from build123d import *

# Parameters (mm, degrees)
SKETCH1_R           = 1.5
SKETCH1_W           = 14
SKETCH1_H           = 14
BOSS_EXTRUDE1_DEPTH = 1.6
CUT_EXTRUDE1_DEPTH  = 1.6
FILLET1_R           = 3
SKETCH3_W           = 5.928661094
SKETCH3_H           = 12.435728147
SKETCH3_W_2         = 5.350255133
SKETCH3_H_2         = 5.928661094
SKETCH3_W_3         = 5.639458113
SKETCH3_W_4         = 6.651668543
SKETCH3_H_3         = 7.446976739
SKETCH3_W_5         = 5.928661093
SKETCH3_H_4         = 5.784059603
SKETCH3_H_5         = 4.627247683
BOSS_EXTRUDE2_DEPTH = 1.6
CUT_EXTRUDE2_DEPTH  = 95.202490958
FILLET2_R           = 3
CUT_EXTRUDE3_DEPTH  = 95.202490958
FILLET3_R           = 3
FILLET4_R           = 3
FILLET7_R           = 2


with BuildPart() as part:
    # Sketch1 → Boss-Extrude1 (new body)
    with BuildSketch(Plane.XY):
        with BuildLine():
            Line((69.256483633, 39.154946315), (-80.703110167, 39.058787515))
            ThreePointArc((-80.703110167, 39.058787515), (-82.819785745, 38.18282616), (-83.701171171, 36.068403419))
            Line((-83.701171171, 36.068403419), (-83.931946571, -35.933513481))
            ThreePointArc((-83.931946571, -35.933513481), (-83.056679124, -38.061046878), (-80.931961975, -38.943128786))
            Line((-80.931961975, -38.943128786), (-34.162352475, -38.943128786))
            ThreePointArc((-34.162352475, -38.943128786), (-34.036703471, -38.945761219), (-33.911274976, -38.953653901))
            Line((-33.911274976, -38.953653901), (11.083089424, -42.732603701))
            ThreePointArc((11.083089424, -42.732603701), (11.20851792, -42.740496382), (11.334166924, -42.743128815))
            Line((11.334166924, -42.743128815), (59.596129524, -42.743128815))
            ThreePointArc((59.596129524, -42.743128815), (61.35026035, -42.176855395), (62.442179406, -40.69181219))
            Line((62.442179406, -40.69181219), (72.104457106, -11.70497919))
            ThreePointArc((72.104457106, -11.70497919), (72.219669608, -11.236842575), (72.258407243, -10.756295796))
            Line((72.258407243, -10.756295796), (72.258407243, 36.154946904))
            ThreePointArc((72.258407243, 36.154946904), (71.379047386, 38.276947252), (69.256483633, 39.154946315))
        make_face()
        with Locations((35.108407229, 34.256871219)):
            Circle(SKETCH1_R, mode=Mode.SUBTRACT)
        with Locations((-28.161592771, -22.743128781)):
            Circle(SKETCH1_R, mode=Mode.SUBTRACT)
        with Locations((-1.491592771, -27.493128781)):
            Circle(SKETCH1_R, mode=Mode.SUBTRACT)
        with Locations((-79.366592771, -9.443128781)):
            Circle(SKETCH1_R, mode=Mode.SUBTRACT)
        with Locations((49.358407229, -9.443128781)):
            Circle(SKETCH1_R, mode=Mode.SUBTRACT)
        with Locations((-59.891592771, 17.156871219)):
            Circle(SKETCH1_R, mode=Mode.SUBTRACT)
        with Locations((2.808407229, 28.556871219)):
            Rectangle(SKETCH1_W, SKETCH1_H, mode=Mode.SUBTRACT)
        with Locations((21.808407229, 28.556871219)):
            Rectangle(SKETCH1_W, SKETCH1_H, mode=Mode.SUBTRACT)
        with Locations((-35.191592771, 28.556871219)):
            Rectangle(SKETCH1_W, SKETCH1_H, mode=Mode.SUBTRACT)
        with Locations((-16.191592771, 28.556871219)):
            Rectangle(SKETCH1_W, SKETCH1_H, mode=Mode.SUBTRACT)
        with Locations((-70.816592771, 9.556871219)):
            Rectangle(SKETCH1_W, SKETCH1_H, mode=Mode.SUBTRACT)
        with Locations((-49.441592771, 9.556871219)):
            Rectangle(SKETCH1_W, SKETCH1_H, mode=Mode.SUBTRACT)
        with Locations((-30.441592771, 9.556871219)):
            Rectangle(SKETCH1_W, SKETCH1_H, mode=Mode.SUBTRACT)
        with Locations((-11.441592771, 9.556871219)):
            Rectangle(SKETCH1_W, SKETCH1_H, mode=Mode.SUBTRACT)
        with Locations((-39.941592771, -9.443128781)):
            Rectangle(SKETCH1_W, SKETCH1_H, mode=Mode.SUBTRACT)
        with Locations((-1.941592771, -9.443128781)):
            Rectangle(SKETCH1_W, SKETCH1_H, mode=Mode.SUBTRACT)
        with Locations((26.558407229, 9.556871219)):
            Rectangle(SKETCH1_W, SKETCH1_H, mode=Mode.SUBTRACT)
        with Locations((36.058407229, -9.443128781)):
            Rectangle(SKETCH1_W, SKETCH1_H, mode=Mode.SUBTRACT)
        with Locations((17.508407229, -32.243128781)):
            Rectangle(SKETCH1_W, SKETCH1_H, mode=Mode.SUBTRACT)
        with Locations((-70.816592771, -28.443128781)):
            Rectangle(SKETCH1_W, SKETCH1_H, mode=Mode.SUBTRACT)
        with Locations((-73.191592771, 28.556871219)):
            Rectangle(SKETCH1_W, SKETCH1_H, mode=Mode.SUBTRACT)
        with Locations((-54.191592771, 28.556871219)):
            Rectangle(SKETCH1_W, SKETCH1_H, mode=Mode.SUBTRACT)
        with Locations((7.558407229, 9.556871219)):
            Rectangle(SKETCH1_W, SKETCH1_H, mode=Mode.SUBTRACT)
        with Locations((-66.066592771, -9.443128781)):
            Rectangle(SKETCH1_W, SKETCH1_H, mode=Mode.SUBTRACT)
        with Locations((-20.941592771, -9.443128781)):
            Rectangle(SKETCH1_W, SKETCH1_H, mode=Mode.SUBTRACT)
        with Locations((17.058407229, -9.443128781)):
            Rectangle(SKETCH1_W, SKETCH1_H, mode=Mode.SUBTRACT)
        with Locations((-47.161592771, -28.443128781)):
            Rectangle(SKETCH1_W, SKETCH1_H, mode=Mode.SUBTRACT)
        with Locations((46.508407229, -32.243128781)):
            Rectangle(SKETCH1_W, SKETCH1_H, mode=Mode.SUBTRACT)
    extrude(amount=BOSS_EXTRUDE1_DEPTH)

    # Sketch2 → Cut-Extrude1 (cut)
    with BuildSketch(Plane.XY.offset(1.6)):
        Polygon((39.377336656, 41.971884199), (39.377336656, 0), (47.100744033, 0), (47.100744033, -5.977603272), (56.433194615, -5.977603272), (56.433194615, -45.238257442), (88.453154369, -41.859266714), (93.4411883, 41.971884199), align=None)
    extrude(amount=-CUT_EXTRUDE1_DEPTH, mode=Mode.SUBTRACT)

    # Fillet1
    fillet1_edges = [part.edges().sort_by_distance(p)[0] for p in [
        (56.433194615, -42.743128815, 0.8),
        (39.377336656, 39.135786868, 0.8),
        (56.433194615, -5.977603272, 0.8),
        (47.100744033, 0, 0.8),
    ]]
    fillet(fillet1_edges, radius=FILLET1_R)

    # Sketch3 → Boss-Extrude2 (add, through all)
    with BuildSketch(Plane.XY.offset(1.6)):
        with Locations((-78.603151983, -9.902316574)):
            Rectangle(SKETCH3_W, SKETCH3_H)
        with Locations((-60.094161253, 17.210462816)):
            Rectangle(SKETCH3_W_2, SKETCH3_H_2)
        with Locations((-27.992630455, -23.133352916)):
            Rectangle(SKETCH3_W_3, SKETCH3_H_2)
        with Locations((-1.313655536, -26.856841286)):
            Rectangle(SKETCH3_W_4, SKETCH3_H_3)
        with Locations((49.658369718, -10.480722534)):
            Rectangle(SKETCH3_W_5, SKETCH3_H_4)
        with Locations((35.05361922, 33.911934921)):
            Rectangle(SKETCH3_W_2, SKETCH3_H_5)
    extrude(amount=-BOSS_EXTRUDE2_DEPTH)

    # Sketch4 → Cut-Extrude2 (cut, through all)
    with BuildSketch(Plane.XY.offset(1.6)):
        Polygon((47.100744033, -5.977603272), (47.100744033, -21.90424025), (70.264082054, -21.90424025), (70.264082054, 0), align=None)
    extrude(amount=-CUT_EXTRUDE2_DEPTH, mode=Mode.SUBTRACT)

    # Fillet2
    fillet2_edges = [part.edges().sort_by_distance(p)[0] for p in [
        (56.433194615, -21.90424025, 0.8),
    ]]
    fillet(fillet2_edges, radius=FILLET2_R)

    # Sketch5 → Cut-Extrude3 (cut, through all)
    with BuildSketch(Plane.XY.offset(1.6)):
        Polygon((39.377336656, 20.463996343), (32.089288673, 20.463996343), (32.089288673, 44.034039226), (51.321286853, 44.034039226), align=None)
    extrude(amount=-CUT_EXTRUDE3_DEPTH, mode=Mode.SUBTRACT)

    # Fillet3
    fillet3_edges = [part.edges().sort_by_distance(p)[0] for p in [
        (32.089288673, 39.131113542, 0.8),
    ]]
    fillet(fillet3_edges, radius=FILLET3_R)

    # Fillet4
    fillet4_edges = [part.edges().sort_by_distance(p)[0] for p in [
        (39.377336656, 20.463996343, 0.8),
    ]]
    fillet(fillet4_edges, radius=FILLET4_R)

    # Fillet7
    fillet7_edges = [part.edges().sort_by_distance(p)[0] for p in [
        (39.377336656, 0, 0.8),
        (47.100744033, -21.90424025, 0.8),
        (32.089288673, 20.463996343, 0.8),
    ]]
    fillet(fillet7_edges, radius=FILLET7_R)


solid = part.part
Input: part model. Units: mm. Frame: model coordinates. Coordinates: 2 decimals unless noted, no trailing zeros. Loops run counter-clockwise (first coordinate to the right, second up) from the corner with the lowest first, then second, coordinate; pieces in that order, holes last.
(1) Section D-D on y = -28. Return the cut outline in (x, z), then the cut area to 3 significant figures.
(2) Section B-B on x = -11. Return the cut outline in (y, z), then the cut area to 3 significant figures.
(3) Section A-A on y = 26.5. Return the cut outline in (x, z).
(4) Section C-C on z = 0.3. Count the separate pieces of the cut face and the enclosed holes in it, then the cut area to 3 significant figures.
(5) Material intervals for probe 1 along X at (y, z) = (-34.5, 0.5); probe 2 along Y at (x, z) = (-52, 0.6); probe 3 along Y at (x, z) = (20, 0.65), sorted ascending.
(6) First-contact query: pin 1 Ø0.5 at (x, z) = (-39, 0.5) entering from +Y; pin 2 Ø0.8 at (y, z) = (-7.5, 0.5) entering from +X; pin 3 Ø0.5 at (y, z) = (12.5, 1) entering from +X. Flat tips, straight axial feed; report the tip coordinate or a pass-through.
Data:
1. outline: (-83.91, 0) - (-77.82, 0) - (-77.82, 1.6) - (-83.91, 1.6) - close; (-63.82, 0) - (-54.16, 0) - (-54.16, 1.6) - (-63.82, 1.6) - close; (-40.16, 0) - (10.51, 0) - (10.51, 1.6) - (-40.16, 1.6) - close; (24.51, 0) - (39.51, 0) - (39.51, 1.6) - (24.51, 1.6) - close; (53.51, 0) - (56.43, 0) - (56.43, 1.6) - (53.51, 1.6) - close
1. area: 135 mm2
2. outline: (-40.88, 0) - (2.56, 0) - (2.56, 1.6) - (-40.88, 1.6) - close; (16.56, 0) - (21.56, 0) - (21.56, 1.6) - (16.56, 1.6) - close; (35.56, 0) - (39.1, 0) - (39.1, 1.6) - (35.56, 1.6) - close
2. area: 83.2 mm2
3. outline: (-83.73, 0) - (-80.19, 0) - (-80.19, 1.6) - (-83.73, 1.6) - close; (-66.19, 0) - (-61.19, 0) - (-61.19, 1.6) - (-66.19, 1.6) - close; (-47.19, 0) - (-42.19, 0) - (-42.19, 1.6) - (-47.19, 1.6) - close; (-28.19, 0) - (-23.19, 0) - (-23.19, 1.6) - (-28.19, 1.6) - close; (-9.19, 0) - (-4.19, 0) - (-4.19, 1.6) - (-9.19, 1.6) - close; (9.81, 0) - (14.81, 0) - (14.81, 1.6) - (9.81, 1.6) - close; (28.81, 0) - (32.09, 0) - (32.09, 1.6) - (28.81, 1.6) - close
4. separate pieces: 1
4. enclosed holes: 22
4. area: 5,870 mm2
5. probe 1: x = -83.93 to -77.82, -63.82 to -54.16, -40.16 to 10.51, 24.51 to 39.51, 53.51 to 56.43
5. probe 2: y = -38.94 to -35.44, -21.44 to 2.56, 16.56 to 21.56, 35.56 to 39.08
5. probe 3: y = -42.74 to -39.24, -25.24 to -16.44, -2.44 to 2.56, 16.56 to 21.56, 35.56 to 39.12
6. pin 1: stops at y = 39.09
6. pin 2: stops at x = 47.1
6. pin 3: stops at x = 39.38
